For this review, take the finished solid that the model builds, in its own axes (mm). A direction names the side the tool comes from. Give positions to 0.01 mm unless a question says otherwise; leave off trailing zeros. Write each loop counter-clockwise with the first axis right and the second up, starting at its lowest first coordinate (ties: lowest second). Pieces come first, ordered by that corner, then holes. Notation, with made-up numbers: M 89.5,-28.75 L 142.5,-28.75 A22 ccw 142.5,-9.75 Z; hole C -36.5,85 d10. An arc over 180 degrees is marked long. One line per item, written item: value. Start each with the question number.
Item 1: Consider section D-D, the plane z = 11.5. Write out the cut boundary in (x, y).
Item 2: Clearance check with flat-ended pins moving along their axes: pin 1 Ø4.5 at (y, z) = (30.5, -10) entering from -X; pin 2 Ø3.5 at (y, z) = (5, 18.5) entering from +X; pin 3 Ø1 at (x, z) = (5, 14) entering from +Y. State where each tip first meets the part, or that it passes through.
Item 3: Mouldability with a two-part tool opening along Y and no side actions: class faces 1 (the face through (-1, 0, 0)), 2 (the face through (0, 4, 23)), 3 (the face through (-1.172, 46.923, -9.437)), 4 (the face through (30, 16, 0)) as released by +Y, released by -Y, zero draft, split by the parting line, or undercut.
Item 4: Consider section A-A, the plane x = 0. Write out the cut boundary in (y, z).
Item 5: To check wall thickness, follow probe 1 along Z at (x, y) = (-5.5, 23.5); probe 2 along Y at (x, z) = (18, -10); probe 3 along Y at (x, z) = (0, -11). State the ranges of each line that lie inside material, in increasing order.
Item 6: Consider section C-C, the plane x = 21. Write out the cut boundary in (y, z), and give its area (3 significant figures).
Item 7: Tool access review of faces 5 (the face through (-24, 12, 5)), 6 (the face through (16, 3, 18)), 7 (the face through (16, 27, -9)), 8 (the face through (-31, 8, 14)), 9 (the face through (-16, 27, -9)): name each direction out of +Z, -Z, +X, -X, +Y, -Y from which nothing blocks a thin tool from reaching the whole face with its end or side.
Item 8: Consider section B-B, the plane y = 30. Write out the cut boundary in (x, z).
```python
from build123d import *

# Parameters (mm, degrees)
SKETCH_1_W          = 80
SKETCH_1_H          = 28
EXTRUDE_1_DEPTH     = 16
SKETCH_2_W          = 48
SKETCH_2_H          = 19
CUT_EXTRUDE_1_DEPTH = 9
SKETCH_3_W          = 32
SKETCH_3_H          = 7
EXTRUDE_2_DEPTH     = 9
SKETCH_4_R          = 9
EXTRUDE_3_DEPTH     = 9


with BuildPart() as part:
    # 草图1 → 凸台-拉伸1 (new body)
    with BuildSketch(Plane(origin=(0, 0, 0), x_dir=(1, 0, 0), z_dir=(0, 1, 0))):
        Rectangle(SKETCH_1_W, SKETCH_1_H)
    extrude(amount=EXTRUDE_1_DEPTH)

    # 草图2 → 切除-拉伸1 (cut)
    with BuildSketch(Plane(origin=(0, 16, 0), x_dir=(1, 0, 0), z_dir=(0, 1, 0))):
        with Locations((0, -4.5)):
            Rectangle(SKETCH_2_W, SKETCH_2_H)
    extrude(amount=-CUT_EXTRUDE_1_DEPTH, mode=Mode.SUBTRACT)

    # 草图3 → 凸台-拉伸2 (add)
    with BuildSketch(Plane.XY.offset(14)):
        with Locations((0, 3.5)):
            Rectangle(SKETCH_3_W, SKETCH_3_H)
    extrude(amount=EXTRUDE_2_DEPTH)

    # 草图4 → 凸台-拉伸3 (add)
    with BuildSketch(Plane.XY.offset(-5)):
        with BuildLine():
            Line((-16, 16), (16, 16))
            Line((16, 16), (16, 38))
            ThreePointArc((16, 38), (0, 54), (-16, 38))
            Line((-16, 38), (-16, 16))
        make_face()
        with Locations((0, 38)):
            Circle(SKETCH_4_R, mode=Mode.SUBTRACT)
    extrude(amount=-EXTRUDE_3_DEPTH)


solid = part.part
```
Model answer:
1. outline: M -40,0 L 40,0 L 40,16 L 24,16 L 24,7 L -24,7 L -24,16 L -40,16 Z
2. pin 1: stops at x = -16
2. pin 2: stops at x = 16
2. pin 3: stops at y = 7
3. face 1: released by -Y
3. face 2: zero draft
3. face 3: undercut
3. face 4: released by +Y
4. outline: M 0,-14 L 29,-14 L 29,-5 L 7,-5 L 7,23 L 0,23 Z; M 47,-14 L 54,-14 L 54,-5 L 47,-5 Z
5. probe 1: z = -14 to -5
5. probe 2: y = 0 to 16
5. probe 3: y = 0 to 29, 47 to 54
6. outline: M 0,-14 L 16,-14 L 16,-5 L 7,-5 L 7,14 L 0,14 Z
6. area: 277 mm2
7. face 5: +Z, +Y
7. face 6: +Z, +X, +Y, -Y
7. face 7: +Z, -Z, +X, +Y
7. face 8: +Z, -X, +Y, -Y
7. face 9: +Z, -Z, -X, +Y
8. outline: M -16,-14 L -4.12,-14 L -4.12,-5 L -16,-5 Z; M 4.12,-14 L 16,-14 L 16,-5 L 4.12,-5 Z
